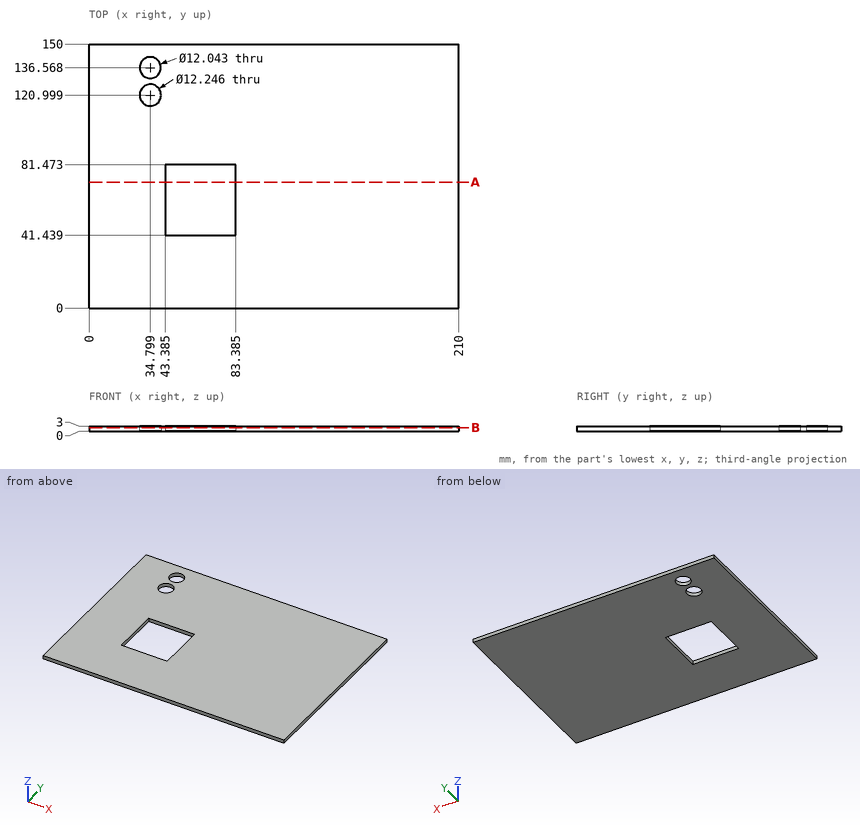
Study the drawing (mm; zero at the part's minimum x, y, z) and answer. Give positions to 0.01 mm unless a question says otherwise; leave off trailing zeros. Write each loop counter-clockwise with the first axis right and the second up, starting at its lowest first coordinate (ties: lowest second). Pieces come first, ordered by that corner, then holes.
(1) The part is cut by section B-B on z = 2.1. Write down the section's boundary in (x, y) (1 decimal).
Final values:
outline: (0, 0) - (210, 0) - (210, 150) - (0, 150) - close; hole circle Ø12.2 at (34.8, 121); hole circle Ø12 at (34.8, 136.6); hole (43.4, 41.4) - (83.4, 41.4) - (83.4, 81.5) - (43.4, 81.5) - close
(2) Straight lines are drawn through the part: line 1 (Y direction, x = 79, z = 0.55); line 2 (X direction, y = 70, z = 0.55) (1 decimal). For each, find the intervals that lie inside material, in ascending order.
Final values:
line 1: y = 0 to 41.44, 81.47 to 150
line 2: x = 0 to 43.4, 83.4 to 210
(3) A flat-ended cylindrical pin translates along its axis: pin 1 Ø11 at (x, y) = (34.8, 136.57) entering from +Z. Find the tip coordinate at first contact, or state that the pin passes through.
Final values:
pin 1: passes through
(4) The part is cut by section A-A on y = 71.5. Write down the section's boundary in (x, z) (1 decimal).
Final values:
outline: (0, 0) - (43.4, 0) - (43.4, 3) - (0, 3) - close; (83.4, 0) - (210, 0) - (210, 3) - (83.4, 3) - close
